Build history of the part. All positions in model axes, mm. Face numbers are marked on the shaded views. A direction names the side the tool comes from. Give positions to 0.01 mm unless a question says otherwise; leave off trailing zeros. Loops run counter-clockwise (first coordinate to the right, second up) from the corner with the lowest first, then second, coordinate; pieces in that order, holes last. Notation, with made-up numbers: (-7.5, 82.25) -> (44.5, 82.25) arc R21 cw to (44.5, 92.25) -> close; hole circle Ø9 at (-29.75, 79). An arc over 180 degrees is marked (long way). Answer in a Markdown table with one row per item. Add a question column.
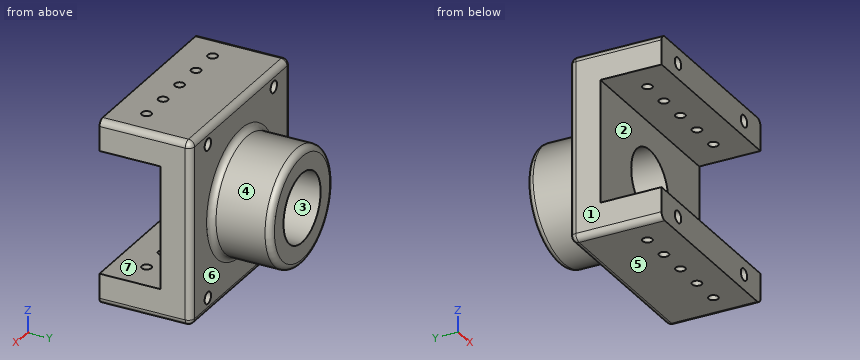
from build123d import *

# Parameters (mm, degrees)
SKETCH2_W                       = 76.2
SKETCH2_H                       = 76.2
SKETCH2_R                       = 14.2875
BOSS_EXTRUDE1_DEPTH             = 12.7
SKETCH3_R                       = 23.8125
SKETCH3_R_2                     = 14.2875
BOSS_EXTRUDE2_DEPTH             = 25.4
SKETCH4_W                       = 76.2
SKETCH4_H                       = 12.7
BOSS_EXTRUDE3_DEPTH             = 25.4
F_10_0_1935_DIAMETER_HOLE1_D    = 4.9149
FILLET1_R                       = 2.54
FILLET2_R                       = 2.54
F_5_32_0_15625_DIAMETER_HOLE1_D = 3.96875


with BuildPart() as part:
    # Sketch2 → Boss-Extrude1 (new body)
    with BuildSketch(Plane(origin=(0, 0, 0), x_dir=(1, 0, 0), z_dir=(0, 1, 0))):
        Rectangle(SKETCH2_W, SKETCH2_H)
        with Locations(Location((0, 0, 0), (0, 0, 270))):
            Circle(SKETCH2_R, mode=Mode.SUBTRACT)
    extrude(amount=BOSS_EXTRUDE1_DEPTH)

    # Sketch3 → Boss-Extrude2 (add)
    with BuildSketch(Plane(origin=(0, 12.7, 0), x_dir=(1, 0, 0), z_dir=(0, 1, 0))):
        with Locations(Location((0, 0, 0), (0, 0, 270))):
            Circle(SKETCH3_R)
        with Locations(Location((0, 0, 0), (0, 0, 270))):
            Circle(SKETCH3_R_2, mode=Mode.SUBTRACT)
    extrude(amount=BOSS_EXTRUDE2_DEPTH)

    # Sketch4 → Boss-Extrude3 (add)
    with BuildSketch(Plane.XZ):
        with Locations((0, -31.75)):
            Rectangle(SKETCH4_W, SKETCH4_H)
        with Locations((0, 31.75)):
            Rectangle(SKETCH4_W, SKETCH4_H)
    extrude(amount=BOSS_EXTRUDE3_DEPTH)

    # #10 (0.1935) Diameter Hole1 (through all)
    with Locations(Plane(origin=(0, -25.4, 0), x_dir=(-1, 0, 0), z_dir=(0, -1, 0))):
        with Locations((-25.4, 31.75), (25.4, 31.75), (25.4, -31.75), (-25.4, -31.75)):
            Hole(F_10_0_1935_DIAMETER_HOLE1_D / 2)

    # Fillet1
    fillet1_edges = [part.edges().sort_by_distance(p)[0] for p in [
        (0, 12.7, -23.8125),
        (0, 38.1, -23.8125),
        (38.1, -6.35, 38.1),
        (-38.1, -6.35, 38.1),
        (-38.1, -6.35, -38.1),
        (38.1, -6.35, -38.1),
    ]]
    fillet(fillet1_edges, radius=FILLET1_R)

    # Fillet2
    fillet2_edges = [part.edges().sort_by_distance(p)[0] for p in [
        (38.1, 12.7, 0),
        (0, 12.7, 38.1),
        (0, 12.7, -38.1),
        (-38.1, 12.7, 0),
        (37.356051224, 12.7, -37.356051224),
        (-37.356051224, 12.7, -37.356051224),
        (-37.356051224, 12.7, 37.356051224),
        (37.356051224, 12.7, 37.356051224),
    ]]
    fillet(fillet2_edges, radius=FILLET2_R)

    # 5/32 (0.15625) Diameter Hole1 (through all)
    with Locations(Plane(origin=(0, 0, -38.1), x_dir=(-1, 0, 0), z_dir=(0, 0, -1))):
        with Locations((0, -12.7), (12.7, -12.7), (25.4, -12.7), (-12.7, -12.7), (-25.4, -12.7)):
            Hole(F_5_32_0_15625_DIAMETER_HOLE1_D / 2)


solid = part.part
(1) Saw through at B-B, the plane x = 0. State how many separate pieces and enclosed holes the cut face has, then the cut area to 3 significant figures.
(2) Saw through at D-D, the plane z = -28. List the corners of the cut face in (x, y).
(3) Saw through at A-A, the plane z = 0. List the corners of the cut face in (x, y), then the cut area to 3 significant figures.
(4) Wall check: line 1 along X through (y, z) = (-13, -31.75); line 2 along Z through (x, y) = (-0.5, -0.5); line 3 along X through (y, z) = (-12, 35). Give the ranges that are in metal, low to high. Write a range as from..to.
(5) Flat gauge pins, fed straight in: pin 1 Ø12 at (y, z) = (25, 0) entering from -X; pin 2 Ø3 at (x, y) = (-25.4, -12.7) entering from +Z (3 decimals); pin 3 Ø12 at (x, y) = (-26.5, 25.5) entering from -Z; pin 4 Ø12 at (x, y) = (-23, 23.5) entering from -Z. Where does each tip first touch, or does it go through?
(6) Two-plate mould, pull along X, no slides. Class the marked faces 1, 2, 3 and 4: released by +X, released by -X, zero draft, split by the parting line, or undercut.
(7) 3-axis set-ups, long thin cutter, end or side, ignore diameter. For the marked faces 5, 6 and 7: which of +Z, -Z, +X, -X, +Y, -Y reach the whole face in a straight line?
Worked answers:
| question | item | result |
|---|---|---|
| 1 | separate pieces | 4 |
| 1 | enclosed holes | 0 |
| 1 | area | 1,630 mm^2 |
| 2 | outline | (-38.1, -25.4) -> (38.1, -25.4) -> (38.1, 10.16) arc R2.54 ccw to (35.56, 12.7) -> (-35.56, 12.7) arc R2.54 ccw to (-38.1, 10.16) -> close; hole circle Ø3.97 at (-25.4, -12.7); hole circle Ø3.97 at (-12.7, -12.7); hole circle Ø3.97 at (0, -12.7); hole circle Ø3.97 at (12.7, -12.7); hole circle Ø3.97 at (25.4, -12.7) |
| 3 | outline | (-38.1, 0) -> (-14.29, 0) -> (-14.29, 38.1) -> (-21.27, 38.1) arc R2.54 ccw to (-23.81, 35.56) -> (-23.81, 15.24) arc R2.54 cw to (-26.35, 12.7) -> (-35.56, 12.7) arc R2.54 ccw to (-38.1, 10.16) -> close; (14.29, 0) -> (38.1, 0) -> (38.1, 10.16) arc R2.54 ccw to (35.56, 12.7) -> (26.35, 12.7) arc R2.54 cw to (23.81, 15.24) -> (23.81, 35.56) arc R2.54 ccw to (21.27, 38.1) -> (14.29, 38.1) -> close |
| 3 | area | 1,090 mm^2 |
| 4 | line 1 | -38.1..-27.86, -22.94..-14.66, -10.74..-1.96, 1.96..10.74, 14.66..22.94, 27.86..38.1 |
| 4 | line 2 | -38.1..-25.4, 25.4..38.1 |
| 4 | line 3 | -38.1..-27.26, -23.54..-14.56, -10.84..-1.86, 1.86..10.84, 14.56..23.54, 27.26..38.1 |
| 5 | pin 1 | x = -23.81 |
| 5 | pin 2 | through |
| 5 | pin 3 | z = -12.12 |
| 5 | pin 4 | z = -16.67 |
| 6 | face 1 | released by -X |
| 6 | face 2 | zero draft |
| 6 | face 3 | undercut |
| 6 | face 4 | split by the parting line |
| 7 | face 5 | -Z, +X, -X, +Y, -Y |
| 7 | face 6 | +Y |
| 7 | face 7 | +X, -X, -Y |
